Check sheet for the modelled part. Datum: model origin and axes. Units: mm. Face numbers are marked on the shaded views. Round coordinates to 2 decimals unless told otherwise and drop trailing zeros. Write each loop counter-clockwise with the first axis right and the second up, starting at its lowest first coordinate (ties: lowest second). Pieces come first, ordered by that corner, then holes. Notation, with made-up numbers: (45, 81) - (99, 81) arc R37 ccw to (99, 119) - close; hole circle Ø4 at (6, 65.25). An arc over 180 degrees is marked (long way). Use one line per item in the form item = value. Start each with the question number.
1) Section check C-C (x = -9). Count the separate pieces of the cut face and the enclosed holes in it, then the cut area to 3 significant figures.
2) Gauge pin test, flat ends, axial feed: P1, Ø2, axis at y = 4, z = -15.5, coming from the -X side; P2, Ø1.5, axis at x = -27.5, y = 1.5, coming from the -Z side; P3, Ø2, axis at y = 3, z = -26.5, coming from the +X side. Record the tip position at first contact, or that the pin passes through.
3) Section check B-B (x = 0). Record the boundary of the cut face in (y, z).
4) Draft check along Z on the marked faces 1, 2 and 3. Enter one of: +Z half, -Z half, draft (parallel to the pull), parting line (faces both ways), or undercut.
5) Scan lines: probe 1 along Z at (x, y) = (-10.5, 4.2); probe 2 along X at (y, z) = (4.3, 13); probe 3 along Z at (x, y) = (26.5, 0.45). Record each from-to range of solid material in increasing order.
6) Section check A-A (z = 0). Record the boundary of the cut face in (x, y).
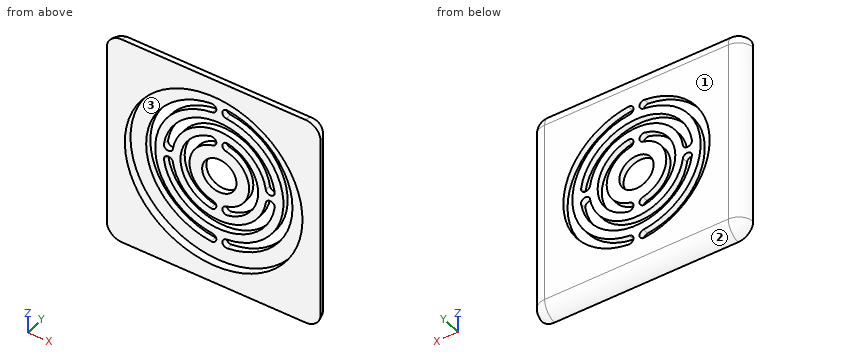
from build123d import *

# Parameters (mm, degrees)
EXTRUDE_1_DEPTH     = 4.7
FILLET_1_R          = 5
SKETCH_2_R          = 29.5
CUT_EXTRUDE_1_DEPTH = 2.7
SKETCH_3_R          = 5.7
CUT_EXTRUDE_2_DEPTH = 51.42410138


with BuildPart() as part:
    # Эскиз1 → Бобышка-Вытянуть1 (new body)
    with BuildSketch(Plane(origin=(0, 0, 0), x_dir=(1, 0, 0), z_dir=(0, 1, 0))):
        with BuildLine():
            Line((-30.5, 35.5), (30.5, 35.5))
            ThreePointArc((30.5, 35.5), (34.035533906, 34.035533906), (35.5, 30.5))
            Line((35.5, 30.5), (35.5, -30.5))
            ThreePointArc((35.5, -30.5), (34.035533906, -34.035533906), (30.5, -35.5))
            Line((30.5, -35.5), (-30.5, -35.5))
            ThreePointArc((-30.5, -35.5), (-34.035533906, -34.035533906), (-35.5, -30.5))
            Line((-35.5, -30.5), (-35.5, 30.5))
            ThreePointArc((-35.5, 30.5), (-34.035533906, 34.035533906), (-30.5, 35.5))
        make_face()
    extrude(amount=EXTRUDE_1_DEPTH)

    # Скругление1
    # the kernel refuses this fillet: 5 mm, written as the material it takes off along each edge
    with BuildSketch(Plane(origin=(-30.5, 4.7, 30.5), x_dir=(0, 0, 1), z_dir=(1, 0, 0))) as fillet_1_piece_1:
        with BuildLine():
            CenterArc((0.009008115, 5), FILLET_1_R, 270, 86.560187232)
            Line((0.009008115, 0), (0.009008115, -0.1))
            Line((0.009008115, -0.1), (5, -0.1))
            Line((5, -0.1), (5.1, 0))
            ThreePointArc((5.1, 0), (5.1, 2.35), (5.099819838, 4.694))
            Line((5.099819838, 4.694), (5, 4.7))
        make_face()
    revolve(axis=Axis((-30.5, 4.7, 30.5), (0, -1, 0)), revolution_arc=90, mode=Mode.SUBTRACT)
    with BuildSketch(Plane(origin=(-35.5, 4.7, 30.5), x_dir=(0, -1, 0), z_dir=(0, 0, -1)), Plane(origin=(-30.5, 4.7, -35.5), x_dir=(0, -1, 0), z_dir=(1, 0, 0)), Plane(origin=(35.5, 4.7, -30.5), x_dir=(0, -1, 0), z_dir=(0, 0, 1)), Plane(origin=(30.5, 4.7, 35.5), x_dir=(0, -1, 0), z_dir=(-1, 0, 0))) as fillet_1_piece_2:
        with BuildLine():
            CenterArc((5, -4.990991885), FILLET_1_R, 93.439812768, 86.560187232)
            Line((0, -4.990991885), (-0.1, -4.990991885))
            Line((-0.1, -4.990991885), (-0.1, 0))
            Line((-0.1, 0), (0, 0.1))
            ThreePointArc((0, 0.1), (2.35, 0.1), (4.694, 0.099819838))
            Line((4.694, 0.099819838), (4.7, 0))
        make_face()
    extrude(amount=61, mode=Mode.SUBTRACT)
    with BuildSketch(Plane(origin=(-30.5, 4.7, -30.5), x_dir=(-1, 0, 0), z_dir=(0, 0, 1))) as fillet_1_piece_3:
        with BuildLine():
            CenterArc((0.009008115, 5), FILLET_1_R, 270, 86.560187232)
            Line((0.009008115, 0), (0.009008115, -0.1))
            Line((0.009008115, -0.1), (5, -0.1))
            Line((5, -0.1), (5.1, 0))
            ThreePointArc((5.1, 0), (5.1, 2.35), (5.099819838, 4.694))
            Line((5.099819838, 4.694), (5, 4.7))
        make_face()
    revolve(axis=Axis((-30.5, 4.7, -30.5), (0, -1, 0)), revolution_arc=90, mode=Mode.SUBTRACT)
    with BuildSketch(Plane(origin=(30.5, 4.7, -30.5), x_dir=(0, 0, -1), z_dir=(-1, 0, 0))) as fillet_1_piece_4:
        with BuildLine():
            CenterArc((0.009008115, 5), FILLET_1_R, 270, 86.560187232)
            Line((0.009008115, 0), (0.009008115, -0.1))
            Line((0.009008115, -0.1), (5, -0.1))
            Line((5, -0.1), (5.1, 0))
            ThreePointArc((5.1, 0), (5.1, 2.35), (5.099819838, 4.694))
            Line((5.099819838, 4.694), (5, 4.7))
        make_face()
    revolve(axis=Axis((30.5, 4.7, -30.5), (0, -1, 0)), revolution_arc=90, mode=Mode.SUBTRACT)
    with BuildSketch(Plane(origin=(30.5, 4.7, 30.5), x_dir=(1, 0, 0), z_dir=(0, 0, -1))) as fillet_1_piece_5:
        with BuildLine():
            CenterArc((0.009008115, 5), FILLET_1_R, 270, 86.560187232)
            Line((0.009008115, 0), (0.009008115, -0.1))
            Line((0.009008115, -0.1), (5, -0.1))
            Line((5, -0.1), (5.1, 0))
            ThreePointArc((5.1, 0), (5.1, 2.35), (5.099819838, 4.694))
            Line((5.099819838, 4.694), (5, 4.7))
        make_face()
    revolve(axis=Axis((30.5, 4.7, 30.5), (0, -1, 0)), revolution_arc=90, mode=Mode.SUBTRACT)

    # Эскиз2 → Вырез-Вытянуть1 (cut)
    with BuildSketch(Plane(origin=(0, 0, 0), x_dir=(1, 0, 0), z_dir=(0, 1, 0))):
        with Locations(Location((0, 0, 0), (0, 0, 90))):
            Circle(SKETCH_2_R)
    extrude(amount=CUT_EXTRUDE_1_DEPTH, mode=Mode.SUBTRACT)

    # Эскиз3 → Вырез-Вытянуть2 (cut, through all)
    with BuildSketch(Plane(origin=(0, 4.7, 0), x_dir=(1, 0, 0), z_dir=(0, 1, 0))):
        with Locations(Location((0, 0, 0), (0, 0, 270))):
            Circle(SKETCH_3_R)
        with BuildLine():
            ThreePointArc((2.828947368, -12.585986524), (12.9, 0), (2.828947368, 12.585986524))
            ThreePointArc((2.828947368, 12.585986524), (1.036513195, 11.451447087), (2.171052632, 9.659012914))
            ThreePointArc((2.171052632, 9.659012914), (9.9, 0), (2.171052632, -9.659012914))
            ThreePointArc((2.171052632, -9.659012914), (1.036513195, -11.451447087), (2.828947368, -12.585986524))
        make_face()
        with BuildLine():
            ThreePointArc((-2.828947368, 12.585986524), (-12.9, 0), (-2.828947368, -12.585986524))
            ThreePointArc((-2.828947368, -12.585986524), (-1.036513195, -11.451447087), (-2.171052632, -9.659012914))
            ThreePointArc((-2.171052632, -9.659012914), (-9.9, 0), (-2.171052632, 9.659012914))
            ThreePointArc((-2.171052632, 9.659012914), (-1.036513195, 11.451447087), (-2.828947368, 12.585986524))
        make_face()
        with BuildLine():
            ThreePointArc((18.400147202, 2.719298246), (0, 18.6), (-18.400147202, 2.719298246))
            ThreePointArc((-18.400147202, 2.719298246), (-17.135562609, 1.016117161), (-15.432381524, 2.280701754))
            ThreePointArc((-15.432381524, 2.280701754), (0, 15.6), (15.432381524, 2.280701754))
            ThreePointArc((15.432381524, 2.280701754), (17.135562609, 1.016117161), (18.400147202, 2.719298246))
        make_face()
        with BuildLine():
            ThreePointArc((-18.400147202, -2.719298246), (0, -18.6), (18.400147202, -2.719298246))
            ThreePointArc((18.400147202, -2.719298246), (17.135562609, -1.016117161), (15.432381524, -2.280701754))
            ThreePointArc((15.432381524, -2.280701754), (0, -15.6), (-15.432381524, -2.280701754))
            ThreePointArc((-15.432381524, -2.280701754), (-17.135562609, -1.016117161), (-18.400147202, -2.719298246))
        make_face()
        with BuildLine():
            ThreePointArc((-2.664473684, 24.153479666), (-24.3, 0), (-2.664473684, -24.153479666))
            ThreePointArc((-2.664473684, -24.153479666), (-1.009044465, -22.826997815), (-2.335526316, -21.171568596))
            ThreePointArc((-2.335526316, -21.171568596), (-21.3, 0), (-2.335526316, 21.171568596))
            ThreePointArc((-2.335526316, 21.171568596), (-1.009044465, 22.826997815), (-2.664473684, 24.153479666))
        make_face()
        with BuildLine():
            ThreePointArc((2.664473684, -24.153479666), (24.3, 0), (2.664473684, 24.153479666))
            ThreePointArc((2.664473684, 24.153479666), (1.009044465, 22.826997815), (2.335526316, 21.171568596))
            ThreePointArc((2.335526316, 21.171568596), (21.3, 0), (2.335526316, -21.171568596))
            ThreePointArc((2.335526316, -21.171568596), (1.009044465, -22.826997815), (2.664473684, -24.153479666))
        make_face()
    extrude(amount=-CUT_EXTRUDE_2_DEPTH, mode=Mode.SUBTRACT)


solid = part.part
Results are:
q1.separate_pieces = 7
q1.enclosed_holes = 0
q1.area = 124 mm²
q2.P1 = -34.27
q2.P2 = -35.4
q2.P3 = 34.95
q3.outline = (0, -35.5) arc R5 ccw to (4.7, -30.51) - (4.7, -18.6) - (2.7, -18.6) - (2.7, -29.5) - (0, -29.5) - close; (0, 29.5) - (2.7, 29.5) - (2.7, 18.6) - (4.7, 18.6) - (4.7, 30.51) arc R5 ccw to (0, 35.5) - close; (2.7, -15.6) - (4.7, -15.6) - (4.7, -5.7) - (2.7, -5.7) - close; (2.7, 5.7) - (4.7, 5.7) - (4.7, 15.6) - (2.7, 15.6) - close
q4.face_1 = draft
q4.face_2 = -Z half
q4.face_3 = undercut
q5.probe_1 = -32.69 to -21.91, -18.53 to -15.35, -11.54 to -7.49, 7.49 to 11.54, 15.35 to 18.53, 21.91 to 32.69
q5.probe_2 = -32.47 to -20.53, -16.87 to -13.3, -8.62 to 8.62, 13.3 to 16.87, 20.53 to 32.47
q5.probe_3 = -35.45 to -12.96, 12.96 to 35.45
q6.outline = (-35.5, 0) - (-29.5, 0) - (-29.5, 2.7) - (-24.3, 2.7) - (-24.3, 4.7) - (-30.51, 4.7) arc R5 ccw to start; (-21.3, 2.7) - (-12.9, 2.7) - (-12.9, 4.7) - (-21.3, 4.7) - close; (-9.9, 2.7) - (-5.7, 2.7) - (-5.7, 4.7) - (-9.9, 4.7) - close; (5.7, 2.7) - (9.9, 2.7) - (9.9, 4.7) - (5.7, 4.7) - close; (12.9, 2.7) - (21.3, 2.7) - (21.3, 4.7) - (12.9, 4.7) - close; (24.3, 2.7) - (29.5, 2.7) - (29.5, 0) - (35.5, 0) arc R5 ccw to (30.51, 4.7) - (24.3, 4.7) - close
